```python
from build123d import *

# Parameters (mm, degrees)
F1_DEPTH = 63.5
F2_DEPTH = 25.4
F3_DEPTH = 7.9375
F4_DEPTH = 25.4
F5_R     = 6.35


with BuildPart() as f1:
    # F0 (on Front) → F1 (new body, symmetric)
    with BuildSketch(Plane.XZ):
        Polygon((22.225, 9.525), (-41.275, 9.525), (-41.275, -9.525), (41.275, -9.525), (41.275, 9.525), align=None)
    extrude(amount=F1_DEPTH, both=True)

    # F0 (on Front) → F2 (join, symmetric)
    with BuildSketch(Plane.XZ):
        with BuildLine():
            Line((22.225, 32.177767), (22.225, 9.525))
            Line((22.225, 9.525), (41.275, 9.525))
            Line((41.275, 9.525), (41.275, 32.177767))
            ThreePointArc((41.275, 32.177767), (44.408206, 39.741994), (51.972433, 42.8752))
            Line((51.972433, 42.8752), (60.325, 42.8752))
            Line((60.325, 42.8752), (60.325, 61.9252))
            Line((60.325, 61.9252), (51.972433, 61.9252))
            ThreePointArc((51.972433, 61.9252), (30.937821, 53.212379), (22.225, 32.177767))
        make_face()
        Polygon((60.325, 66.675), (60.325, 61.9252), (60.325, 42.8752), (85.725, 42.8752), (85.725, 66.675), align=None)
    extrude(amount=F2_DEPTH, both=True)

    # F0 (on Front) → F3 (join, symmetric)
    with BuildSketch(Plane.XZ):
        with BuildLine():
            add(Edge.make_bspline(
                [(-41.275, 9.525), (-17.174726, 36.691695), (14.035416, 64.275697), (51.972433, 61.9252)],
                knots=[0, 0, 0, 0, 106.961978, 106.961978, 106.961978, 106.961978], degree=3))
            Line((-41.275, 9.525), (22.225, 9.525))
            Line((22.225, 9.525), (22.225, 32.177767))
            ThreePointArc((22.225, 32.177767), (30.937821, 53.212379), (51.972433, 61.9252))
        make_face()
    extrude(amount=F3_DEPTH, both=True)

    # F0 (on Front) → F4 (join, symmetric)
    with BuildSketch(Plane.XZ):
        Polygon((111.125, 66.675), (85.725, 66.675), (85.725, 42.8752), (85.725, 38.1), (111.125, 38.1), align=None)
    extrude(amount=F4_DEPTH, both=True)

    # F5
    f5_edges = [f1.edges().sort_by_distance(p)[0] for p in [
        (-41.275, -63.5, 0),
        (41.275, -63.5, 0),
        (-41.275, 63.5, 0),
        (41.275, 63.5, 0),
    ]]
    fillet(f5_edges, radius=F5_R)


solid = f1.part
```
Design review of the part built by this model. Coordinates are the model's own, in mm. A direction names the side the tool comes from. Give positions to 0.01 mm unless a question says otherwise; leave off trailing zeros. Loops run counter-clockwise (first coordinate to the right, second up) from the corner with the lowest first, then second, coordinate; pieces in that order, holes last. Notation, with made-up numbers: (-29.5, 34.5) -> (17.5, 34.5) arc R15 ccw to (17.5, 46.5) -> close; hole circle Ø10 at (46, 18). An arc over 180 degrees is marked (long way). One line per item, written item: value.
Q1. Machinability: for faces 5 (the flat face through (66, 25.4, 45)), 6 (the flat face through (69, 0, 42.875)), 7 (the flat face through (6, -7.938, 31)), 8 (the cylindrical face through (31.17, 16.55, 53.44)), 9 (the flat face through (66, -25.4, 45)), which of the approach directions +Z, -Z, +X, -X, +Y, -Y give a long, thin tool a straight path to every point of the face, cutting with its end or side? Answer none if there is none.
Numbers:
face 5: +Z, +X, -X, +Y
face 6: -Z, +Y, -Y
face 7: +Z, -X, -Y
face 8: +Z, -X, +Y
face 9: +Z, +X, -X, -Y
Q2. For pin 1 Ø4 at (y, z) = (7.5, 40) entering from -X; pin 2 Ø19 at (y, z) = (21, 23) entering from -X (3 decimals); pin 3 Ø6 at (x, z) = (19, 48.5) entering from -Y, all flat-tipped, find the tip position at first contact; note any pin that passes through.
Numbers:
pin 1: stops at x = -12.02
pin 2: stops at x = 22.225
pin 3: stops at y = -7.94
Q3. We need section A-A on z = 7. Give the boundary of the cut face in (x, y) (3 decimals), and give its area (3 significant figures).
Numbers:
outline: (-41.275, -57.15) arc R6.35 ccw to (-34.925, -63.5) -> (34.925, -63.5) arc R6.35 ccw to (41.275, -57.15) -> (41.275, 57.15) arc R6.35 ccw to (34.925, 63.5) -> (-34.925, 63.5) arc R6.35 ccw to (-41.275, 57.15) -> close
area: 10,400 mm^2
Q4. For L1, parallel to Z at x = 40, y = 43 (3 decimals); L2, parallel to Y at x = 17, z = 14; L3, parallel to X at y = 9, z = 8 (3 decimals), list the stretches that pass through material, from the lowest coordinate up.
Numbers:
L1: z = -9.525 to 9.525
L2: y = -7.94 to 7.94
L3: x = -41.275 to 41.275
Q5. We need section D-D on x = 76. Give the boundary of the cut face in (y, z) (3 decimals), and give its area (3 significant figures).
Numbers:
outline: (-25.4, 42.875) -> (25.4, 42.875) -> (25.4, 66.675) -> (-25.4, 66.675) -> close
area: 1,210 mm^2
Q6. Draft analysis for pull direction X (two halves, no side actions). For faces 1 (the flat face through (6, 7.938, 31)), 2 (the flat face through (56, 0, 61.925)), 3 (the flat face through (22.225, -17, 21)), 4 (the cylindrical face through (44.325, -0.356, 39.658)), state which applies: pulls with the +X half, pulls with the -X half, needs draft (parallel to the pull), parting line crosses it, or undercut.
Numbers:
face 1: needs draft
face 2: undercut
face 3: pulls with the -X half
face 4: undercut
Q7. We need section C-C on x = 101.5. Give the boundary of the cut face in (y, z) (3 decimals).
Numbers:
outline: (-25.4, 38.1) -> (25.4, 38.1) -> (25.4, 66.675) -> (-25.4, 66.675) -> close
Q8. We need section B-B on y = -18. Give the boundary of the cut face in (x, z) (3 decimals), and give its area (3 significant figures).
Numbers:
outline: (-41.275, -9.525) -> (41.275, -9.525) -> (41.275, 32.178) arc R10.697 cw to (51.972, 42.875) -> (85.725, 42.875) -> (85.725, 38.1) -> (111.125, 38.1) -> (111.125, 66.675) -> (60.325, 66.675) -> (60.325, 61.925) -> (51.972, 61.925) arc R29.747 ccw to (22.225, 32.178) -> (22.225, 9.525) -> (-41.275, 9.525) -> close
area: 4,100 mm^2
